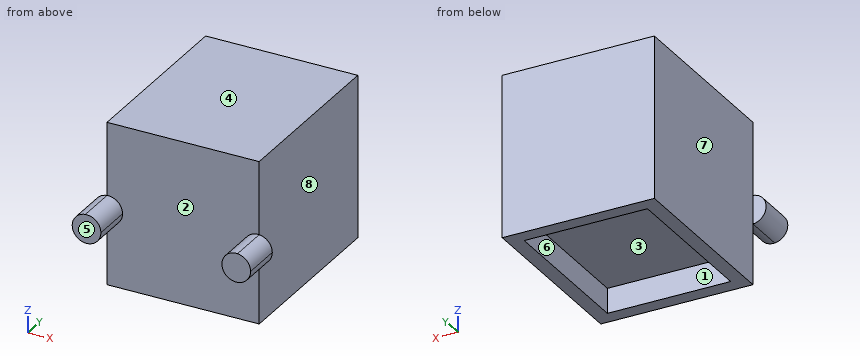
from build123d import *

# Parameters (mm, degrees)
BOSS_EXTRUDE1_DEPTH = 3.2
SKETCH1_3_W         = 12.2
SKETCH1_3_H         = 13
BOSS_EXTRUDE2_DEPTH = 14.55
CUT_EXTRUDE1_START  = -6
SKETCH2_W           = 9.87658836
SKETCH2_H           = 12.271413297
CUT_EXTRUDE1_DEPTH  = 2


with BuildPart() as part:
    # Sketch1 → Boss-Extrude1 (new body)
    with BuildSketch(Plane(origin=(0, 0, 0), x_dir=(1, 0, 0), z_dir=(0, 1, 0))):
        with BuildLine():
            ThreePointArc((-4.85, 0), (-5.222986487, 0.847791248), (-6.1, 1.145643924))
            Line((-6.1, 1.145643924), (-6.1, -1.145643924))
            ThreePointArc((-6.1, -1.145643924), (-5.222986487, -0.847791248), (-4.85, 0))
        make_face()
        with BuildLine():
            Line((-6.1, -1.145643924), (-6.1, 1.145643924))
            ThreePointArc((-6.1, 1.145643924), (-7.15, 0), (-6.1, -1.145643924))
        make_face()
        with BuildLine():
            ThreePointArc((7.15, 0), (6.847791248, 0.777013513), (6.1, 1.145643924))
            Line((6.1, 1.145643924), (6.1, -1.145643924))
            ThreePointArc((6.1, -1.145643924), (6.847791248, -0.777013513), (7.15, 0))
        make_face()
        with BuildLine():
            Line((6.1, -1.145643924), (6.1, 1.145643924))
            ThreePointArc((6.1, 1.145643924), (4.85, 0), (6.1, -1.145643924))
        make_face()
    extrude(amount=-BOSS_EXTRUDE1_DEPTH)

    # Sketch1<3> → Boss-Extrude2 (add)
    with BuildSketch(Plane(origin=(0, 0, 0), x_dir=(1, 0, 0), z_dir=(0, 1, 0))):
        with Locations((0, -0.5)):
            Rectangle(SKETCH1_3_W, SKETCH1_3_H)
    extrude(amount=BOSS_EXTRUDE2_DEPTH)

    # Sketch2 → Cut-Extrude1 (cut)
    with BuildSketch(Plane.XY.offset(CUT_EXTRUDE1_START)):
        with Locations((0, 7.301829354)):
            Rectangle(SKETCH2_W, SKETCH2_H)
    extrude(amount=CUT_EXTRUDE1_DEPTH, mode=Mode.SUBTRACT)


solid = part.part
Design review of the part built by this model. Coordinates are the model's own, in mm. Face numbers are marked on the shaded views. A direction names the side the tool comes from. Give positions to 0.01 mm unless a question says otherwise; leave off trailing zeros. Order: outer loops, then holes, each group sorted by start corner. A loop starts at its lowest first (then second) coordinate and runs counter-clockwise, first axis right, second up. Notation, with made-up numbers: (56, 10) - (115, 10) arc R19 cw to (115, 27) - close; hole circle Ø6 at (-21.5, 15.25). An arc over 180 degrees is marked (long way). Use CSV: the item, a comma, the result in double quotes. Start each with the question number.
Q1. Take a section at B-B (y = 11). State the section outline as (x, z) points.
Q2. Draft analysis for pull direction Y (two halves, no side actions). For the marked faces 1, 2, 3 and 4, state which applies: pulls with the +Y half, pulls with the -Y half, needs draft (parallel to the pull), parting line crosses it, or undercut.
Q3. Take a section at C-C (z = -1.5). State the section outline as (x, y) points, and give its area (3 significant figures).
Q4. For P1, Ø2, axis at x = 1, z = -4.5, coming from the -Y side; P2, Ø1.5, axis at y = 10, z = -3, coming from the -X side; P3, Ø4, axis at y = 12, z = -2.5, coming from the +X side; P4, Ø8, axis at x = -2, y = 9, coming from the -Z side, all flat-tipped, find the tip position at first contact; note any pin that passes through.
Q5. Take a section at A-A (x = 3.5). State the section outline as (y, z) points.
Q6. Machinability: for the marked faces 5, 6, 7 and 8, which of the approach directions +Z, -Z, +X, -X, +Y, -Y give a long, thin tool a straight path to every point of the face, cutting with its end or side? Answer none if there is none.
Q7. For line 1 (X direction, y = -1.75, z = 0); line 2 (Z direction, x = -1.5, y = 7); line 3 (X direction, y = 5.5, z = 2), list the stretches that pass through material, from the lowest coordinate up.
Calculated:
1,outline,"(-6.1, -6) - (-4.94, -6) - (-4.94, -4) - (4.94, -4) - (4.94, -6) - (6.1, -6) - (6.1, 7) - (-6.1, 7) - close"
2,face 1,"undercut"
2,face 2,"pulls with the -Y half"
2,face 3,"undercut"
2,face 4,"needs draft"
3,outline,"(-6.1, 0) - (6.1, 0) - (6.1, 14.55) - (-6.1, 14.55) - close"
3,area,"178 mm²"
4,P1,"stops at y = 0"
4,P2,"stops at x = -6.1"
4,P3,"stops at x = 6.1"
4,P4,"stops at z = -6"
5,outline,"(0, -6) - (1.17, -6) - (1.17, -4) - (13.44, -4) - (13.44, -6) - (14.55, -6) - (14.55, 7) - (0, 7) - close"
6,face 5,"+Z, -Z, +X, -X, -Y"
6,face 6,"-Z"
6,face 7,"+Z, -Z, -X, +Y"
6,face 8,"+Z, -Z, +X, +Y"
7,line 1,"x = -7.15 to -4.85, 4.85 to 7.15"
7,line 2,"z = -4 to 7"
7,line 3,"x = -6.1 to 6.1"
